from build123d import *

# Parameters (mm, degrees)
SKETCH_1_R               = 2
SKETCH_1_R_2             = 1.35
EXTRUDE_1_DEPTH          = 1.5
EXTRUDE_1_2_DEPTH        = 1.5
EXTRUDE_1_3_DEPTH        = 1.5
EXTRUDE_1_4_DEPTH        = 1.5
EXTRUDE_3_DEPTH          = 1.5
SKETCH_5_R               = 6.5
CUT_EXTRUDE_1_DEPTH      = 15.221462653
EXTRUDE_START            = 2
SKETCH_4_R               = 17
SKETCH_4_R_2             = 6.5
EXTRUDE_4_DEPTH          = 2
CUT_EXTRUDE_4_DEPTH      = 25.124676164
CUT_EXTRUDE_4_DEPTH_BACK = 25.124676164
SKETCH_8_R               = 1.35
SKETCH_6_W               = 8
SKETCH_6_H               = 5
CUT_EXTRUDE_2_DEPTH      = 25.124676164
CUT_EXTRUDE_3_DEPTH      = 25.124676164
CUT_EXTRUDE_5_DEPTH      = 24.963513933
FILLET_1_R               = 2
FILLET_2_R               = 1


with BuildPart() as part:
    # Sketch 1 → Extrude 1 (new body)
    with BuildSketch(Plane(origin=(0, 0, 0), x_dir=(1, 0, 0), z_dir=(0, 1, 0))):
        with Locations(Location((0, 8, 0), (0, 0, 270))):
            Circle(SKETCH_1_R)
        with Locations(Location((0, 8, 0), (0, 0, 270))):
            Circle(SKETCH_1_R_2, mode=Mode.SUBTRACT)
    extrude(amount=EXTRUDE_1_DEPTH)



with BuildPart() as body_2:
    # Sketch 1 → Extrude 1 2 (new body)
    with BuildSketch(Plane(origin=(0, 0, 0), x_dir=(1, 0, 0), z_dir=(0, 1, 0))):
        with Locations(Location((8, 0, 0), (0, 0, 270))):
            Circle(SKETCH_1_R)
        with Locations(Location((8, 0, 0), (0, 0, 270))):
            Circle(SKETCH_1_R_2, mode=Mode.SUBTRACT)
    extrude(amount=EXTRUDE_1_2_DEPTH)


with BuildPart() as body_3:
    # Sketch 1 → Extrude 1 3 (new body)
    with BuildSketch(Plane(origin=(0, 0, 0), x_dir=(1, 0, 0), z_dir=(0, 1, 0))):
        with Locations(Location((0, -8, 0), (0, 0, 270))):
            Circle(SKETCH_1_R)
        with Locations(Location((0, -8, 0), (0, 0, 270))):
            Circle(SKETCH_1_R_2, mode=Mode.SUBTRACT)
    extrude(amount=EXTRUDE_1_3_DEPTH)


with BuildPart() as body_4:
    # Sketch 1 → Extrude 1 4 (new body)
    with BuildSketch(Plane(origin=(0, 0, 0), x_dir=(1, 0, 0), z_dir=(0, 1, 0))):
        with Locations(Location((-8, 0, 0), (0, 0, 270))):
            Circle(SKETCH_1_R)
        with Locations(Location((-8, 0, 0), (0, 0, 270))):
            Circle(SKETCH_1_R_2, mode=Mode.SUBTRACT)
    extrude(amount=EXTRUDE_1_4_DEPTH)


with BuildPart() as part_1:
    add(part.part)

    add(body_2.part)  # Extrude 3 merges body 2

    add(body_3.part)  # Extrude 3 merges body 3

    add(body_4.part)  # Extrude 3 merges body 4
    # Sketch 3 → Extrude 3 (add)
    with BuildSketch(Plane.XZ):
        with BuildLine():
            ThreePointArc((-1.414213562, -9.414213562), (-2, -8), (-1.414213562, -6.585786438))
            Line((-1.414213562, -6.585786438), (-6.585786438, -1.414213562))
            ThreePointArc((-6.585786438, -1.414213562), (-8, -2), (-9.414213562, -1.414213562))
            Line((-9.414213562, -1.414213562), (-1.414213562, -9.414213562))
        make_face()
        with BuildLine():
            Line((-1.414213562, 9.414213562), (-9.414213562, 1.414213562))
            ThreePointArc((-9.414213562, 1.414213562), (-8, 2), (-6.585786438, 1.414213562))
            Line((-6.585786438, 1.414213562), (-1.414213562, 6.585786438))
            ThreePointArc((-1.414213562, 6.585786438), (-2, 8), (-1.414213562, 9.414213562))
        make_face()
        with BuildLine():
            ThreePointArc((9.414213562, 1.414213562), (8, 2), (6.585786438, 1.414213562))
            Line((6.585786438, 1.414213562), (1.414213562, 6.585786438))
            ThreePointArc((1.414213562, 6.585786438), (2, 8), (1.414213562, 9.414213562))
            Line((1.414213562, 9.414213562), (9.414213562, 1.414213562))
        make_face()
        with BuildLine():
            ThreePointArc((1.414213562, -9.414213562), (2, -8), (1.414213562, -6.585786438))
            Line((1.414213562, -6.585786438), (6.585786438, -1.414213562))
            ThreePointArc((6.585786438, -1.414213562), (8, -2), (9.414213562, -1.414213562))
            Line((9.414213562, -1.414213562), (1.414213562, -9.414213562))
        make_face()
    extrude(amount=-EXTRUDE_3_DEPTH)

    # Sketch 5 → Cut-Extrude 1 (cut, through all)
    with BuildSketch(Plane.XZ):
        Circle(SKETCH_5_R)
    extrude(amount=-CUT_EXTRUDE_1_DEPTH, mode=Mode.SUBTRACT)

    # Sketch 4 → Extrude 4 (add)
    with BuildSketch(Plane.XZ.offset(EXTRUDE_START)):
        with Locations(Location((0, 0, 0), (0, 0, 270))):
            Circle(SKETCH_4_R)
        with Locations(Location((0, 0, 0), (0, 0, 270))):
            Circle(SKETCH_4_R_2, mode=Mode.SUBTRACT)
    extrude(amount=-EXTRUDE_4_DEPTH)

    # Sketch 8 → Cut-Extrude 4 (cut, two sides: drawn at the far end of the back side and taken through both)
    with BuildSketch(Plane(origin=(0, 0, 0), x_dir=(1, 0, 0), z_dir=(0, 1, 0)).offset(-CUT_EXTRUDE_4_DEPTH_BACK)):
        with Locations(Location((8, 0, 0), (0, 0, 270))):
            Circle(SKETCH_8_R)
        with Locations(Location((0, -8, 0), (0, 0, 270))):
            Circle(SKETCH_8_R)
        with Locations(Location((-8, 0, 0), (0, 0, 270))):
            Circle(SKETCH_8_R)
        with Locations(Location((0, 8, 0), (0, 0, 270))):
            Circle(SKETCH_8_R)
    extrude(amount=CUT_EXTRUDE_4_DEPTH + CUT_EXTRUDE_4_DEPTH_BACK, mode=Mode.SUBTRACT)

    # Sketch 6 → Cut-Extrude 2 (cut, through all)
    with BuildSketch(Plane(origin=(0, 0, 0), x_dir=(1, 0, 0), z_dir=(0, 1, 0))):
        with Locations((0, 14.5)):
            Rectangle(SKETCH_6_W, SKETCH_6_H)
    extrude(amount=-CUT_EXTRUDE_2_DEPTH, mode=Mode.SUBTRACT)

    # Sketch 7 → Cut-Extrude 3 (cut, through all)
    with BuildSketch(Plane(origin=(0, 0, 0), x_dir=(1, 0, 0), z_dir=(0, 1, 0))):
        with BuildLine():
            Line((7.392057511, -8.809511096), (10.927389365, -13.022755533))
            ThreePointArc((10.927389365, -13.022755533), (1.924454634, -16.890721547), (-7.717838496, -15.147110911))
            Line((-7.717838496, -15.147110911), (-5.220890747, -10.246575028))
            ThreePointArc((-5.220890747, -10.246575028), (1.301836958, -11.42607634), (7.392057511, -8.809511096))
        make_face()
    extrude(amount=-CUT_EXTRUDE_3_DEPTH, mode=Mode.SUBTRACT)

    # Sketch 11 → Cut-Extrude 5 (cut, through all)
    with BuildSketch(Plane(origin=(0, 1.5, 0), x_dir=(1, 0, 0), z_dir=(0, 1, 0))):
        with BuildLine():
            Line((-8.059965436, 1.348667545), (-6.585786438, 1.414213562))
            Line((-6.585786438, 1.414213562), (-6.263846285, 1.736153715))
            ThreePointArc((-6.263846285, 1.736153715), (-4.596194078, 4.596194078), (-1.736153715, 6.263846285))
            Line((-1.736153715, 6.263846285), (-1.414213562, 6.585786438))
            Line((-1.414213562, 6.585786438), (-1.348667545, 8.059965436))
            ThreePointArc((-1.348667545, 8.059965436), (0, 9.35), (1.348667545, 8.059965436))
            Line((1.348667545, 8.059965436), (1.414213562, 6.585786438))
            Line((1.414213562, 6.585786438), (1.736153715, 6.263846285))
            ThreePointArc((1.736153715, 6.263846285), (4.596194078, 4.596194078), (6.263846285, 1.736153715))
            Line((6.263846285, 1.736153715), (6.585786438, 1.414213562))
            Line((6.585786438, 1.414213562), (8.059965436, 1.348667545))
            ThreePointArc((8.059965436, 1.348667545), (9.35, 0), (8.059965436, -1.348667545))
            Line((8.059965436, -1.348667545), (6.585786438, -1.414213562))
            Line((6.585786438, -1.414213562), (6.263846285, -1.736153715))
            ThreePointArc((6.263846285, -1.736153715), (4.596194078, -4.596194078), (1.736153715, -6.263846285))
            Line((1.736153715, -6.263846285), (1.414213562, -6.585786438))
            Line((1.414213562, -6.585786438), (1.348667545, -8.059965436))
            ThreePointArc((1.348667545, -8.059965436), (0, -9.35), (-1.348667545, -8.059965436))
            Line((-1.348667545, -8.059965436), (-1.414213562, -6.585786438))
            Line((-1.414213562, -6.585786438), (-1.736153715, -6.263846285))
            ThreePointArc((-1.736153715, -6.263846285), (-4.596194078, -4.596194078), (-6.263846285, -1.736153715))
            Line((-6.263846285, -1.736153715), (-6.585786438, -1.414213562))
            Line((-6.585786438, -1.414213562), (-8.059965436, -1.348667545))
            ThreePointArc((-8.059965436, -1.348667545), (-9.35, 0), (-8.059965436, 1.348667545))
        make_face()
    extrude(amount=-CUT_EXTRUDE_5_DEPTH, mode=Mode.SUBTRACT)

    # Fillet 1
    fillet_1_edges = [part_1.edges().sort_by_distance(p)[0] for p in [
        (-4, -1, -12),
        (4, -1, -12),
        (-5.220890747, -1, 10.246575028),
        (7.392057511, -1, 8.809511096),
        (10.927389365, -1, 13.022755533),
        (-7.717838496, -1, 15.147110911),
    ]]
    fillet(fillet_1_edges, radius=FILLET_1_R)

    # Fillet 2
    fillet_2_edges = [part_1.edges().sort_by_distance(p)[0] for p in [
        (4, -1, -16.522711642),
        (-4, -1, -16.522711642),
    ]]
    fillet(fillet_2_edges, radius=FILLET_2_R)


solid = part_1.part
The listing builds one solid part. Answer for the finished solid, in the listing's coordinates (mm). A direction names the side the tool comes from. Round coordinates to 2 decimals unless told otherwise and drop trailing zeros. Order: outer loops, then holes, each group sorted by start corner. A loop starts at its lowest first (then second) coordinate and runs counter-clockwise, first axis right, second up. Notation, with made-up numbers: M 16,8 L 53,8 A32 cw 53,39 Z; hole C 81.25,71.5 d9. An arc over 180 degrees is marked long. Answer in a Markdown table with one row per item. Add a question column.
1) Which of the six approach directions +Z, -Z, +X, -X, +Y, -Y give full straight-line access (tool end or side, diameter ignored) to faces 1 (the face through (-4.56, -0.27, 4.63)), 2 (the face through (0, 1, -10)), 3 (the face through (0, 1, 10)), 4 (the face through (-10, 1, 0))?
2) The part is cut by section B-B on x = 0. Determine the outline of the cut face in (y, z).
3) Determine the mould class of faces 5 (the face through (-0.03, -0.27, 9.35)), 6 (the face through (-5.47, 0.74, -5.36)), 7 (the face through (7.352, -1.014, 9.536)) for opening direction Z: pulls with the +Z half, pulls with the -Z half, needs draft (parallel to the pull), parting line crosses it, or undercut.
4) The part is cut by section C-C on z = 5.5. Determine the outline of the cut face in (x, y), plus the area to 3 significant figures.
5) Flat-ended cylindrical pins translate along their axes: pin 1 Ø3 at (x, z) = (-11, -1) entering from +Y; pin 2 Ø8 at (x, z) = (13.5, 8.5) entering from +Y; pin 3 Ø1.3 at (y, z) = (-0.5, -14.5) entering from +X; pin 4 Ø1 at (x, y) = (0.5, -1) entering from -Z. Find the tip coordinate at first contact, or state that the pin passes through.
6) The part is cut by section D-D on x = -12. Determine the outline of the cut face in (y, z), plus the area to 3 significant figures.
7) Consider line 1 along Y through (x, z) = (3, 10); line 2 along Z through (x, y) = (3, -1.75); line 3 along X through (y, z) = (-0.95, -3). Determine where each line is inside the solid, lowest interval first. Write a range as from..to.
Findings below:
| question | item | result |
|---|---|---|
| 1 | face 1 | +Y, -Y |
| 1 | face 2 | -Z, +Y |
| 1 | face 3 | +Z, +Y |
| 1 | face 4 | -X, +Y |
| 2 | outline | M -2,-12 L 0,-12 L 0,-10 L 1.5,-10 L 1.5,-9.35 L -2,-9.35 Z; M -2,9.35 L 1.5,9.35 L 1.5,10 L 0,10 L 0,11.5 L -2,11.5 Z |
| 3 | face 5 | undercut |
| 3 | face 6 | pulls with the -Z half |
| 3 | face 7 | pulls with the +Z half |
| 4 | outline | M -16.09,-2 L -3.46,-2 L -3.46,1.5 L -5.33,1.5 L -5.33,0 L -16.09,0 Z; M 3.46,-2 L 16.09,-2 L 16.09,0 L 5.33,0 L 5.33,1.5 L 3.46,1.5 Z |
| 4 | area | 56.1 mm² |
| 5 | pin 1 | stops at y = 1.5 |
| 5 | pin 2 | stops at y = 0 |
| 5 | pin 3 | stops at x = 9.86 |
| 5 | pin 4 | stops at z = -12 |
| 6 | outline | M -2,-12.04 L 0,-12.04 L 0,12.04 L -2,12.04 Z |
| 6 | area | 48.2 mm² |
| 7 | line 1 | y = -2..0 |
| 7 | line 2 | z = -12.27..-5.77, 5.77..11.1 |
| 7 | line 3 | x = -16.73..-5.77, 5.77..16.73 |
